```python
from build123d import *

# Parameters (mm, degrees)
SKETCH_AS_DRAWN_R                 = 2
SKETCH_AS_DRAWN_R_2               = 10
SKETCH_AS_DRAWN_R_3               = 1.6
EXTRUDE001_DEPTH                  = 3
EXTRUDE001_ONTO_SKETCH_ROLL_ANGLE = 90


with BuildPart() as part:
    # Sketch as drawn → Extrude001 (new)
    with BuildSketch(Plane.XY):
        with BuildLine():
            ThreePointArc((-48.5, 0), (-46.742641, -4.242641), (-42.5, -6))
            Line((-42.5, -6), (-20.493903, -6))
            ThreePointArc((-18.63082, -7.272727), (-19.36575, -6.348554), (-20.493903, -6))
            ThreePointArc((-18.63082, -7.272727), (0, -20), (18.63082, -7.272727))
            ThreePointArc((20.493902, -6), (19.365749, -6.348554), (18.63082, -7.272727))
            Line((47.5, -6), (20.493902, -6))
            Line((47.5, -6), (47.5, 20))
            Line((47.5, 20), (37, 20))
            ThreePointArc((32, 20), (34.5, 17.5), (37, 20))
            Line((-48.5, 20), (32, 20))
            Line((-48.5, 20), (-48.5, 0))
        make_face()
        with Locations((-42.5, 0)):
            Circle(SKETCH_AS_DRAWN_R, mode=Mode.SUBTRACT)
        Circle(SKETCH_AS_DRAWN_R_2, mode=Mode.SUBTRACT)
        with Locations((-12.124, 7.000616)):
            Circle(SKETCH_AS_DRAWN_R_3, mode=Mode.SUBTRACT)
        with Locations((0, -14)):
            Circle(SKETCH_AS_DRAWN_R_3, mode=Mode.SUBTRACT)
        with Locations((12.124, 7.000616)):
            Circle(SKETCH_AS_DRAWN_R_3, mode=Mode.SUBTRACT)
    extrude(amount=-EXTRUDE001_DEPTH)


with BuildPart() as part_1:
    # Extrude001 onto Sketch roll: moved
    add(part.part.rotate(Axis((0, 0, 0), (1, 0, 0)), EXTRUDE001_ONTO_SKETCH_ROLL_ANGLE))


with BuildPart() as part_2:
    # Extrude001 onto Sketch placement: moved
    add(part_1.part)


solid = part_2.part
```
Part model, mm, in its own coordinate system. A direction names the side the tool comes from. Coordinates: 2 decimals unless noted, no trailing zeros. Loops run counter-clockwise (first coordinate to the right, second up) from the corner with the lowest first, then second, coordinate; pieces in that order, holes last. Notation, with made-up numbers: (19, -32.5) - (53, -32.5) arc R20 ccw to (53, -4.5) - close; hole circle Ø7 at (46.25, 11). An arc over 180 degrees is marked (long way). Write item = value, one per line. Start each with the question number.
Item 1: Mould opens along Z. For faces 1 (the flat face through (-48.5, 1, 10)), 2 (the cylindrical face through (-19.35, 1.48, -6.36)), 3 (the cylindrical face through (11.916, 1.479, 8.587)) say: released by +Z, released by -Z, zero draft, split by the parting line, or undercut.
Item 2: Cut at B-B, the plane z = -14. Give the cut face in (x, y), and give its area (3 significant figures).
Item 3: 3-axis set-ups, long thin cutter, end or side, ignore diameter. For faces 4 (the flat face through (34, 1, -6)), 5 (the flat face through (-32, 1, -6)), 6 (the flat face through (42, 1, 20)): which of +Z, -Z, +X, -X, +Y, -Y reach the whole face in a straight line?
Item 4: Cut at C-C, the plane y = 2.35. Give the cut face in (x, z), and give its area (3 significant figures).
Item 5: Cut at D-D, the plane x = -12. Give the cut face in (y, z), and give its area (3 significant figures).
Item 6: Flat gauge pins, fed straight in: pin 1 Ø5 at (x, z) = (2.5, 5.5) entering from +Y; pin 2 Ø1 at (x, y) = (-31.5, 1.5) entering from -Z. Where does each tip first touch, or does it go through?
Item 7: Cut at A-A, the plane x = 0. Give the cut face in (y, z).
Item 8: Wall check: L1, parallel to Z at x = 0, y = 1.25; L2, parallel to Z at x = -42.5, y = 1.75; L3, parallel to X at y = 1.9, z = 7. Give the ranges that are in metal, low to high. Write a range as from..to.
The answers:
q1.face_1 = zero draft
q1.face_2 = released by -Z
q1.face_3 = undercut
q2.outline = (-14.28, 0) - (-1.6, 0) - (-1.6, 3) - (-14.28, 3) - close; (1.6, 0) - (14.28, 0) - (14.28, 3) - (1.6, 3) - close
q2.area = 76.1 mm2
q3.face_4 = -Z, +X, +Y, -Y
q3.face_5 = -Z, -X, +Y, -Y
q3.face_6 = +Z, +X, -X, +Y, -Y
q4.outline = (-48.5, 0) arc R6 ccw to (-42.5, -6) - (-20.49, -6) arc R2 cw to (-18.63, -7.27) arc R20 ccw to (18.63, -7.27) arc R2 cw to (20.49, -6) - (47.5, -6) - (47.5, 20) - (37, 20) arc R2.5 cw to (32, 20) - (-48.5, 20) - close; hole circle Ø4 at (-42.5, 0); hole circle Ø3.2 at (-12.12, 7); hole circle Ø20 at (0, 0); hole circle Ø3.2 at (0, -14); hole circle Ø3.2 at (12.12, 7)
q4.area = 2,520 mm2
q5.outline = (0, -16) - (3, -16) - (3, 5.41) - (0, 5.41) - close; (0, 8.6) - (3, 8.6) - (3, 20) - (0, 20) - close
q5.area = 98.4 mm2
q6.pin_1 = through
q6.pin_2 = -6
q7.outline = (0, -20) - (3, -20) - (3, -15.6) - (0, -15.6) - close; (0, -12.4) - (3, -12.4) - (3, -10) - (0, -10) - close; (0, 10) - (3, 10) - (3, 20) - (0, 20) - close
q8.L1 = -20..-15.6, -12.4..-10, 10..20
q8.L2 = -6..-2, 2..20
q8.L3 = -48.5..-13.72, -10.52..-7.14, 7.14..10.52, 13.72..47.5
